The listing builds one solid part. Answer for the finished solid, in the listing's coordinates (mm). A direction names the side the tool comes from. Coordinates: 2 decimals unless noted, no trailing zeros. Order: outer loops, then holes, each group sorted by start corner. A loop starts at its lowest first (then second) coordinate and runs counter-clockwise, first axis right, second up. Notation, with made-up numbers: (24, 2) - (34, 2) arc R16 ccw to (34, 28) - close; hole circle Ø5 at (8, 67). An arc over 180 degrees is marked (long way). Use one line per item in the form item = value. Start each with the question number.
Item 1: Section A-A, the plane x = 10.5 is taken. Write down the section's boundary in (y, z).
Item 2: The mould has two halves that part along Y. Classify faces 4 (the flat face through (-4, -1, 2)), 5 (the cylindrical face through (8, -3, 0)), 6 (the flat face through (-2.433, -1.014, -1.724)): released by +Y, released by -Y, zero draft, split by the parting line, or undercut.
Item 3: Consider line 1 along Y through (x, z) = (-2.25, -1.5); line 2 along X through (y, z) = (0, 3.5); line 3 along Z through (x, y) = (2, 0). Determine where each line is inside the solid, lowest interval first. Write a range as [from, to].
Item 4: Each of these flat-tipped pins is pushed along its axis until it touches: pin 1 Ø5 at (x, z) = (11.5, 2) entering from -Y; pin 2 Ø3 at (x, z) = (9, 1) entering from +Y; pin 3 Ø1.5 at (x, z) = (8.5, -3.5) entering from +Y. Where does it stop, or does it pass through?
Item 5: A tool of negligible diameter and unlimited length cuts with its end or side. For faces 1 (the flat face through (0, 3.3, 0.1)), 2 (the flat face through (16, 0, 0)), 3 (the flat face through (-2.43, -0.99, 1.74)), from which of +Z, -Z, +X, -X, +Y, -Y can it reach the whole face along a straight path? Write none if from no direction.
Autodesk Inventor part; units mm, degrees
ref_plane "Work Plane1" through (29, 0, 0) normal (0, -1, 0) x (1, 0, 0)
ref_plane "YZ Plane" through (0, 0, 0) normal (1, 0, 0) x (0, 1, 0)
ref_plane "XZ Plane" through (0, 0, 0) normal (0, 1, 0) x (-1, 0, 0)
sketch "Sketch1" plane through (0, 0, 0) normal (0, 0, 1) x (1, 0, 0)
  line L0 (0.3333, 0) -> (16, 0)
  line L1 (16, 0) -> (16, 3)
  line L2 (16, 3) -> (3, 3)
  line L3 (3, 3) -> (2.3864, 3)
  line L4 (2.3864, 3) -> (0, 3)
  line L5 (0, 3) -> (0, 5)
  line L6 (0, 5) -> (-4, 5)
  line L7 (-4, 5) -> (-4, 2.3094)
  line L8 (-4, 2.3094) -> (-1, 2.3094)
  line L9 (-1, 2.3094) -> (0.3333, 0)
  line L10 (-8, 0) -> (20, 0)
  line L11 (0, -1) -> (0, 6)
  line L12 (3, 3) -> (0, 3) construction
  dimension "d1" = 13
  dimension "d2" = 0.6136
  dimension "d3" = 4
  dimension "d4" = 3
  dimension "d5" = 60
  dimension "d6" = 6
  dimension "d7" = 6
  dimension "d8" = 4.6188
  dimension "d9" = 10
  dimension "d26" = 16
revolve "Body" add sketch "Sketch1" angle 360 about axis through (0.3333, 0, 0) along (1, 0, 0) contours L9 L11 L4 L3 L2 L1 L0 | L9 L8 L7 L6 L5 L11
sketch "Sketch2" plane through (-4, 0, 0) normal (-1, 0, 0) x (0, 0, 1)
  circle A0 centre (0, 0) radius 2.3094
  line L0 (0, -7) -> (0, 7)
  line L1 (-7, 0) -> (7, 0)
  line L2 (2.3094, 0) -> (1.1547, -2)
  line L3 (1.1547, -2) -> (-1.1547, -2)
  line L4 (-1.1547, -2) -> (-2.3094, 0)
  line L5 (-2.3094, 0) -> (-1.1547, 2)
  line L6 (-1.1547, 2) -> (1.1547, 2)
  line L7 (1.1547, 2) -> (2.3094, 0)
extrude "Slot" add sketch "Sketch2" against normal up to next contours L7 A0 | A0 L2 | L6 L0 A0 | A0 L0 L3 | L0 L6 A0 | A0 L3 L0 | L4 A0 | A0 L5
fillet "Fillet1" radius 0.6 1 edges at (-4, -5, 0)
thread "Thread"
chamfer "Chamfer1" distance 0.6135 distance2 0.6135 1 edges at (16, -3, 0) measured on face at (16, -1.1424, 0.935)
ref_plane "Work Plane1" through (29, 0, 0) normal (0, -1, 0) x (1, 0, 0)
fillet "Fillet2" radius 0.1 1 edges at (0, -3, 0)
equation "\"d1\" = GEL"
equation "\"d3\" = KOH"
equation "\"d4\" = INTI"
equation "\"d6\" = GD"
equation "\"d7\" = BDM"
equation "\"d8\" = 1.1547 * SW"
equation "\"d9\" = KOD"
equation "\"d26\" = NLG"
equation "\"d30\" = R"
equation "\"d17\" = RR"
equation "\"d13\" = GEL"
equation "\"d15\" = -0.5 * SPD + 0.5 * GD"
equation "\"d16\" = GUL"
equation "\"GD\" = NND"
equation "\"NLG\" = 16"
equation "\"GEL\" = 13"
equation "\"KOD\" = 10"
equation "\"KOH\" = 4"
equation "\"INTI\" = 3"
equation "\"GAL\" = 0.61345 * PTC"
equation "\"GUL\" = 0.61345 * PTC"
equation "\"BDM\" = NND"
equation "\"SW\" = 4"
equation "\"RR\" = 0.6"
equation "\"SPD\" = NND - 1.2269 * PTC"
equation "\"R\" = 0.1"
equation "\"TOA\" = 30deg"
equation "\"GD1\" = THREADDIA - 1.2269 * PTC"
equation "\"THREADDIA\" = 6"
equation "\"FAWI\" = 45deg"
equation "\"ANG\" = 120deg"
equation "\"PTC\" = 1"
equation "\"NND\" = 6"
equation "\"E0\" = 1.155 * SW"
properties part number "DIN 7984 - M6 x 16" material "Steel, Mild"
Response:
q1.outline = circle Ø6 at (0, 0)
q2.face_4 = zero draft
q2.face_5 = split by the parting line
q2.face_6 = undercut
q3.line_1 = [-4.77, -1.4], [1.4, 4.77]
q3.line_2 = [-4, 0]
q3.line_3 = [-3, 3]
q4.pin_1 = -3
q4.pin_2 = 3
q4.pin_3 = 1.2
q5.face_1 = +X
q5.face_2 = +Z, -Z, +X, +Y, -Y
q5.face_3 = -X
